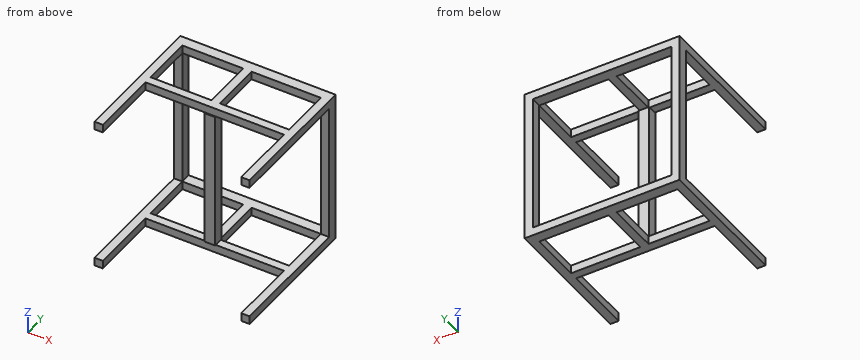
```python
from build123d import *

# Parameters (mm, degrees)
SKETCH1_W           = 300
SKETCH1_H           = 300
SKETCH1_W_2         = 268
SKETCH1_H_2         = 268
BOSS_EXTRUDE1_DEPTH = 20
SKETCH3_W           = 16
SKETCH3_H           = 100
BOSS_EXTRUDE2_DEPTH = 16
SKETCH4_W           = 16
SKETCH4_H           = 250
BOSS_EXTRUDE3_DEPTH = 16
SKETCH5_W           = 268
SKETCH5_H           = 16
BOSS_EXTRUDE4_DEPTH = 16
SKETCH6_W           = 20
SKETCH6_H           = 20
BOSS_EXTRUDE5_DEPTH = 268


with BuildPart() as part:
    # Sketch1 → Boss-Extrude1 (new body)
    with BuildSketch(Plane(origin=(0, 0, 0), x_dir=(1, 0, 0), z_dir=(0, 1, 0))):
        Rectangle(SKETCH1_W, SKETCH1_H)
        Rectangle(SKETCH1_W_2, SKETCH1_H_2, mode=Mode.SUBTRACT)
    extrude(amount=BOSS_EXTRUDE1_DEPTH)

    # Sketch3 → Boss-Extrude2 (add)
    with BuildSketch(Plane.XY.offset(150)):
        with Locations((-8, -50)):
            Rectangle(SKETCH3_W, SKETCH3_H)
    boss_extrude2 = extrude(amount=-BOSS_EXTRUDE2_DEPTH)

    # Sketch4 → Boss-Extrude3 (add)
    with BuildSketch(Plane.XY.offset(150)):
        with Locations((-142, -125)):
            Rectangle(SKETCH4_W, SKETCH4_H)
        with Locations((142, -125)):
            Rectangle(SKETCH4_W, SKETCH4_H)
    boss_extrude3 = extrude(amount=-BOSS_EXTRUDE3_DEPTH)

    # Sketch5 → Boss-Extrude4 (add)
    with BuildSketch(Plane.XY.offset(150)):
        with Locations((0, -108)):
            Rectangle(SKETCH5_W, SKETCH5_H)
    boss_extrude4 = extrude(amount=-BOSS_EXTRUDE4_DEPTH)

    # Mirror1: Boss-Extrude2, Boss-Extrude3, Boss-Extrude4 across plane
    add(boss_extrude2.mirror(Plane.XY))
    add(boss_extrude3.mirror(Plane.XY))
    add(boss_extrude4.mirror(Plane.XY))

    # Sketch6 → Boss-Extrude5 (add)
    with BuildSketch(Plane(origin=(0, 0, 134), x_dir=(-1, 0, 0), z_dir=(0, 0, -1))):
        with Locations((8, -108)):
            Rectangle(SKETCH6_W, SKETCH6_H)
    extrude(amount=BOSS_EXTRUDE5_DEPTH)


solid = part.part
```
Can you work these out from the model? Positions are in its coordinate system, mm. Round coordinates to 2 decimals unless told otherwise and drop trailing zeros. Loops run counter-clockwise (first coordinate to the right, second up) from the corner with the lowest first, then second, coordinate; pieces in that order, holes last.
Item 1: Suppose I cut it at C-C, the plane x = 28.5. Write out the boundary of the cut face in (y, z).
Item 2: Please list where this line runs through material, in increasing order: L1, parallel to X at y = -210, z = 138.
Item 3: Suppose I cut it at D-D, the plane y = -53. Write out the boundary of the cut face in (x, z), then the cut area to 3 significant figures.
Item 4: Will these pins go through, and if not, where does the flat tip stop? pin 1 Ø0.6 at (x, y) = (0.5, -99.5) entering from -Z; pin 2 Ø1.5 at (y, z) = (-114, -25.5) entering from -X; pin 3 Ø6 at (x, z) = (-8, 18.5) entering from +Y.
Item 5: Suppose I cut it at B-B, the plane y = -219. Write out the boundary of the cut face in (x, z), then the cut area to 3 significant figures.
Item 6: Suppose I cut it at A-A, the plane z = 26. Write out the boundary of the cut face in (x, y).
Reported:
1. outline: (-116, -150) - (-100, -150) - (-100, -134) - (-116, -134) - close; (-116, 134) - (-100, 134) - (-100, 150) - (-116, 150) - close; (0, -150) - (20, -150) - (20, -134) - (0, -134) - close; (0, 134) - (20, 134) - (20, 150) - (0, 150) - close
2. L1: x = -150 to -134, 134 to 150
3. outline: (-150, -150) - (-134, -150) - (-134, -134) - (-150, -134) - close; (-150, 134) - (-134, 134) - (-134, 150) - (-150, 150) - close; (-16, -150) - (0, -150) - (0, -134) - (-16, -134) - close; (-16, 134) - (0, 134) - (0, 150) - (-16, 150) - close; (134, -150) - (150, -150) - (150, -134) - (134, -134) - close; (134, 134) - (150, 134) - (150, 150) - (134, 150) - close
3. area: 1,540 mm2
4. pin 1: stops at z = -134
4. pin 2: stops at x = -18
4. pin 3: stops at y = -98
5. outline: (-150, -150) - (-134, -150) - (-134, -134) - (-150, -134) - close; (-150, 134) - (-134, 134) - (-134, 150) - (-150, 150) - close; (134, -150) - (150, -150) - (150, -134) - (134, -134) - close; (134, 134) - (150, 134) - (150, 150) - (134, 150) - close
5. area: 1,020 mm2
6. outline: (-150, 0) - (-134, 0) - (-134, 20) - (-150, 20) - close; (-18, -118) - (2, -118) - (2, -98) - (-18, -98) - close; (134, 0) - (150, 0) - (150, 20) - (134, 20) - close
